Autodesk Inventor part; units mm, degrees
ref_plane "Work Plane1" through (29, 0, 0) normal (0, -1, 0) x (1, 0, 0)
ref_plane "YZ Plane" through (0, 0, 0) normal (1, 0, 0) x (0, 1, 0)
ref_plane "XZ Plane" through (0, 0, 0) normal (0, 1, 0) x (-1, 0, 0)
sketch "Sketch1" plane through (0, 0, 0) normal (0, 0, 1) x (1, 0, 0)
  line L0 (-1.7103, 0) -> (44.45, 0)
  line L1 (44.45, 0) -> (44.45, 3.175)
  line L2 (44.45, 3.175) -> (12.7, 3.175)
  line L3 (12.7, 3.175) -> (9.5249, 3.175)
  line L4 (9.5249, 3.175) -> (0, 3.175)
  line L5 (0, 3.175) -> (0, 4.7625)
  line L6 (0, 4.7625) -> (-6.35, 4.7625)
  line L7 (-6.35, 4.7625) -> (-6.35, 2.757)
  line L8 (-6.35, 2.757) -> (-3.302, 2.757)
  line L9 (-3.302, 2.757) -> (-1.7103, 0)
  line L10 (-16.51, 0) -> (54.61, 0)
  line L11 (0, -0.9525) -> (0, 5.715)
  line L12 (12.7, 3.175) -> (0, 3.175) construction
  dimension "d1" = 31.75
  dimension "d2" = 3.1751
  dimension "d3" = 6.35
  dimension "d4" = 3.048
  dimension "d5" = 60
  dimension "d6" = 6.35
  dimension "d7" = 6.35
  dimension "d8" = 5.5139
  dimension "d9" = 9.525
  dimension "d26" = 44.45
revolve "Body" add sketch "Sketch1" angle 360 about axis through (-1.7103, 0, 0) along (1, 0, 0)
sketch "Sketch2" plane through (-6.35, 0, 0) normal (-1, 0, 0) x (0, 0, 1)
  circle A0 centre (0, 0) radius 2.757
  line L0 (0, -6.6675) -> (0, 6.6675)
  line L1 (-6.6675, 0) -> (6.6675, 0)
  line L2 (2.757, 0) -> (1.3785, -2.3876)
  line L3 (1.3785, -2.3876) -> (-1.3785, -2.3876)
  line L4 (-1.3785, -2.3876) -> (-2.757, 0)
  line L5 (-2.757, 0) -> (-1.3785, 2.3876)
  line L6 (-1.3785, 2.3876) -> (1.3785, 2.3876)
  line L7 (1.3785, 2.3876) -> (2.757, 0)
extrude "Slot" add sketch "Sketch2" against normal up to next contours L7 A0 | A0 L2 | L6 L0 A0 | A0 L0 L3 | L0 L6 A0 | A0 L3 L0 | L4 A0 | A0 L5
fillet "Fillet1" radius 0.635 1 edges at (-6.35, -4.7625, 0)
thread "Thread"
chamfer "Chamfer1" distance 0.7556 distance2 0.7556 1 edges at (44.45, -3.175, 0) measured on face at (44.45, 0.6012, -0.3644)
ref_plane "Work Plane1" through (29, 0, 0) normal (0, -1, 0) x (1, 0, 0)
fillet "Fillet2" radius 0.1778 1 edges at (0, -3.175, 0)
equation "\"d1\" = GEL"
equation "\"d3\" = KOH"
equation "\"d4\" = INTI"
equation "\"d6\" = GD"
equation "\"d7\" = BDM"
equation "\"d8\" = 1.1547 * SW"
equation "\"d9\" = KOD"
equation "\"d26\" = NLG"
equation "\"d30\" = R"
equation "\"d17\" = RR"
equation "\"d13\" = GEL"
equation "\"d15\" = -0.5 * SPD + 0.5 * GD"
equation "\"d16\" = GUL"
equation "\"GD\" = 6.35"
equation "\"NLG\" = 44.45"
equation "\"GEL\" = 31.75"
equation "\"KOD\" = 9.525"
equation "\"KOH\" = 6.35"
equation "\"INTI\" = 3.048"
equation "\"GAL\" = 3.175"
equation "\"GUL\" = 0.75565"
equation "\"BDM\" = 6.35"
equation "\"SW\" = 4.7752"
equation "\"RR\" = 0.635"
equation "\"SPD\" = 4.8387"
equation "\"R\" = 0.1778"
equation "\"PHH\" = 0.2032"
equation "\"GD1\" = SPD"
equation "\"THREADDIA\" = 6.35"
equation "\"FAWI\" = 45deg"
equation "\"KOH1\" = 5.715"
equation "\"NND\" = 6.35"
equation "\"TOA\" = 30deg"
equation "\"E0\" = 1.155 * SW"
properties part number "am-1058" material "Steel, Mild"
Check sheet for the modelled part. Datum: model origin and axes. Units: mm. A direction names the side the tool comes from. Round coordinates to 2 decimals unless told otherwise and drop trailing zeros. Loops run counter-clockwise (first coordinate to the right, second up) from the corner with the lowest first, then second, coordinate; pieces in that order, holes last. Notation, with made-up numbers: (33, 33.5) - (54, 33.5) arc R19 cw to (54, 58.5) - close; hole circle Ø7 at (12.25, -7.75). An arc over 180 degrees is marked (long way). Write item = value, one per line. Start each with the question number.
Q1. Section check A-A (x = 9). Record the boundary of the cut face in (y, z) (3 decimals).
Q2. Release check for a two-part mould opening along Z. For faces 4 (the face through (-2.9, -3.78, 2.9)), 5 (the face through (-6.35, -2, 2)), 6 (the face through (-1.81, 0.165, -0.052)) record: pulls with the +Z half, pulls with the -Z half, needs draft (parallel to the pull), parting line crosses it, or undercut.
Q3. Access from +Z, -Z, +X, -X, +Y, -Y to the whole of each face (thin tool, end or side, straight path). Record for faces 1 (the face through (21.63, -0.69, 3.1)), 2 (the face through (-5, 2.388, 0)), 3 (the face through (44.45, 0, 0)).
Q4. Thickness scan on L1, parallel to X at y = -0.5, z = -4; L2, parallel to Z at x = 22.5, y = 0.25; L3, parallel to Z at x = -3, y = -1.5. Record the ranges inside material, lowest first.
Q5. Depth check by flat-ended pin: P1, Ø1, axis at x = 22, z = -2, coming from the +Y side; P2, Ø1.5, axis at x = 16, z = -1.5, coming from the +Y side; P3, Ø1, axis at x = 13.5, y = -3, coming from the +Z side. Enter the tip coordinate at first touch or a pass-through.
Derived:
q1.outline = circle Ø6.35 at (0, 0)
q2.face_4 = parting line crosses it
q2.face_5 = needs draft
q2.face_6 = undercut
q3.face_1 = +X
q3.face_2 = -X
q3.face_3 = +Z, -Z, +X, +Y, -Y
q4.L1 = -6.35 to 0
q4.L2 = -3.17 to 3.17
q4.L3 = -4.52 to -1.66, 1.66 to 4.52
q5.P1 = 2.8
q5.P2 = 3.09
q5.P3 = 1.96
